Could you check a few things on this drawing? It's one solid part, dimensions in mm from its lowest x, y, z. A direction names the side the tool comes from. Give positions to 0.01 mm unless a question says otherwise; leave off trailing zeros. Order: outer loops, then holes, each group sorted by start corner. A loop starts at its lowest first (then second) coordinate and runs counter-clockwise, first axis right, second up. Notation, with made-up numbers: M 9.25,54.25 L 52.25,54.25 A17 ccw 52.25,58.25 Z; hole C 21.5,-3 d5. An arc over 180 degrees is marked long. One line per item, written item: value. Start each with the question number.
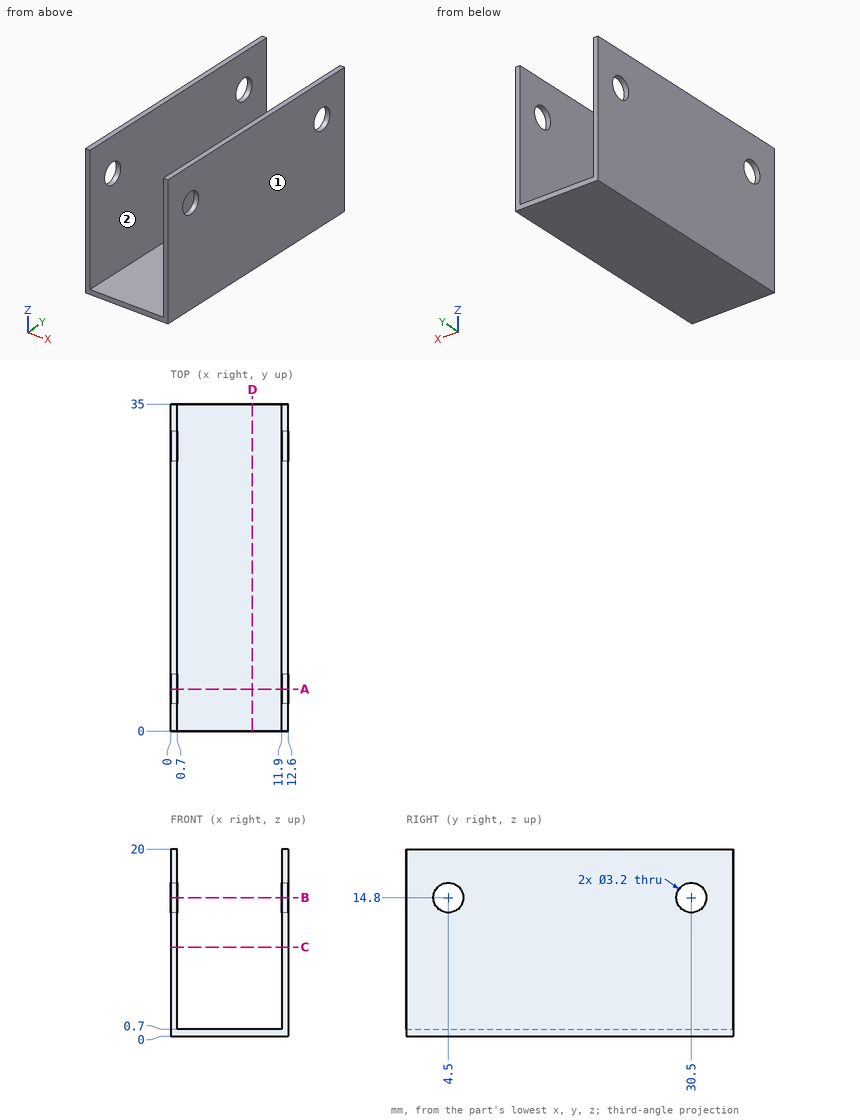
Item 1: Will this pin go through, and if not, where does the flat tip stop? P1, Ø3.5, axis at x = 7, y = 11.5, coming from the +Z side.
Item 2: I want a section at A-A on y = 4.5. Write out the boundary of the cut face in (x, z), plus the area to 3 significant figures.
Item 3: For the marked faces 1 and 2, which set-ups out of +Z, -Z, +X, -X, +Y, -Y let a thin tool reach every point of the face, with its end or its side?
Item 4: I want a section at C-C on z = 9.5. Write out the boundary of the cut face in (x, y).
Item 5: Please list where these lines run through material, in increasing order: probe 1 along X at (y, z) = (9, 11.5); probe 2 along Y at (x, z) = (12.25, 14.8); probe 3 along Z at (x, y) = (4, 10). Write a range as [from, to].
Item 6: I want a section at B-B on z = 14.8. Write out the boundary of the cut face in (x, y).
Item 7: I want a section at D-D on x = 8.75. Write out the boundary of the cut face in (y, z).
Answer below:
1. P1: stops at z = 0.7
2. outline: M 0,0 L 12.6,0 L 12.6,13.2 L 11.9,13.2 L 11.9,0.7 L 0.7,0.7 L 0.7,13.2 L 0,13.2 Z; M 0,16.4 L 0.7,16.4 L 0.7,20 L 0,20 Z; M 11.9,16.4 L 12.6,16.4 L 12.6,20 L 11.9,20 Z
2. area: 31.4 mm²
3. face 1: +Z, -Z, +X, +Y, -Y
3. face 2: +Z, +Y, -Y
4. outline: M 0,0 L 0.7,0 L 0.7,35 L 0,35 Z; M 11.9,0 L 12.6,0 L 12.6,35 L 11.9,35 Z
5. probe 1: x = [0, 0.7], [11.9, 12.6]
5. probe 2: y = [0, 2.9], [6.1, 28.9], [32.1, 35]
5. probe 3: z = [0, 0.7]
6. outline: M 0,0 L 0.7,0 L 0.7,2.9 L 0,2.9 Z; M 0,6.1 L 0.7,6.1 L 0.7,28.9 L 0,28.9 Z; M 0,32.1 L 0.7,32.1 L 0.7,35 L 0,35 Z; M 11.9,0 L 12.6,0 L 12.6,2.9 L 11.9,2.9 Z; M 11.9,6.1 L 12.6,6.1 L 12.6,28.9 L 11.9,28.9 Z; M 11.9,32.1 L 12.6,32.1 L 12.6,35 L 11.9,35 Z
7. outline: M 0,0 L 35,0 L 35,0.7 L 0,0.7 Z
